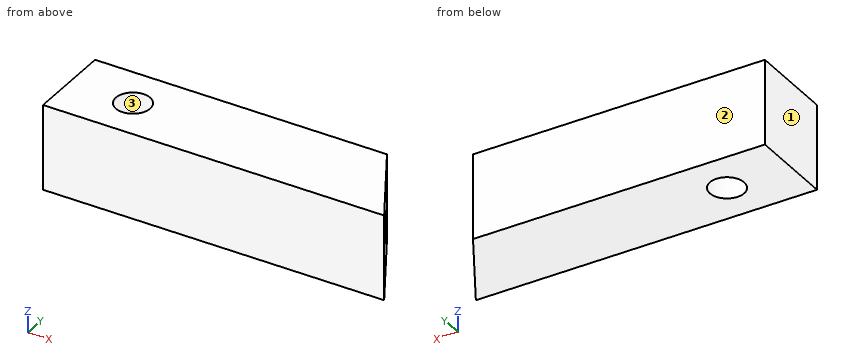
from build123d import *

# Parameters (mm, degrees)
SKETCH1_W                  = 12.7
SKETCH1_H                  = 12.7
BOSS_EXTRUDE1_DEPTH        = 50.8
F_10_32_TAPPED_HOLE1_D     = 4.0386
F_10_32_TAPPED_HOLE1_DEPTH = 25.4
F_10_32_TAPPED_HOLE1_TIP   = 1.213317848
CUT_EXTRUDE1_DEPTH         = 13.7
F_10_CLEARANCE_HOLE1_D     = 5.1054


with BuildPart() as part:
    # Sketch1 → Boss-Extrude1 (new body)
    with BuildSketch(Plane(origin=(0, 0, 0), x_dir=(0, 0, -1), z_dir=(1, 0, 0))):
        with Locations((6.35, 6.35)):
            Rectangle(SKETCH1_W, SKETCH1_H)
    extrude(amount=BOSS_EXTRUDE1_DEPTH)

    # #10-32 Tapped Hole1
    with Locations(Plane(origin=(50.8, 6.35, -6.35), x_dir=(0, 0, 1), z_dir=(1, 0, 0))):
        with Locations((0, 0)):
            Hole(F_10_32_TAPPED_HOLE1_D / 2, depth=F_10_32_TAPPED_HOLE1_DEPTH)
            with Locations((0, 0, -(F_10_32_TAPPED_HOLE1_DEPTH + F_10_32_TAPPED_HOLE1_TIP / 2))):  # 118° drill point
                Cone(0, F_10_32_TAPPED_HOLE1_D / 2, F_10_32_TAPPED_HOLE1_TIP, mode=Mode.SUBTRACT)

    # Sketch3 → Cut-Extrude1 (cut, through all)
    with BuildSketch(Plane.XY):
        Polygon((43.467651581, 12.7), (50.8, 0), (50.8, 12.7), align=None)
    extrude(amount=-CUT_EXTRUDE1_DEPTH, mode=Mode.SUBTRACT)

    # #10 Clearance Hole1 (through all)
    with Locations(Plane(origin=(9.525, 6.35, 0), x_dir=(1, 0, 0), z_dir=(0, 0, 1))):
        with Locations((0, 0)):
            Hole(F_10_CLEARANCE_HOLE1_D / 2)


solid = part.part
Can you work these out from the model? Positions are in its coordinate system, mm. Face numbers are marked on the shaded views. Give positions to 0.01 mm unless a question says otherwise; leave off trailing zeros. Write each loop counter-clockwise with the first axis right and the second up, starting at its lowest first coordinate (ties: lowest second). Pieces come first, ordered by that corner, then holes. Notation, with made-up numbers: (82, 54.25) -> (108, 54.25) arc R12 ccw to (108, 70.25) -> close; hole circle Ø3 at (-8, -6.75). An arc over 180 degrees is marked (long way). Answer as a JSON object with one key per item and string values. Group by question number.
Item 1: Suppose I cut it at C-C (x = 35.5). Please give me the cut outline in (y, z), plus the area to 3 significant figures.
Item 2: Suppose I cut it at A-A (x = 7.5). Please give me the cut outline in (y, z).
Item 3: Please list where these lines run through material, in increasing order: line 1 (Y direction, x = 36, z = -6.35); line 2 (Y direction, x = 28, z = -5); line 3 (Y direction, x = 45.5, z = -2.5). Write a range as [from, to].
Item 4: Suppose I cut it at B-B (z = -3.5). Please give me the cut outline in (x, y) (3 decimals), plus the area to 3 significant figures.
Item 5: I'm going to push a flat-ended pin straight in: P1, Ø3, axis at y = 9.5, z = -5, coming from the +X side. Where does the tip first touch, or does it pass through?
Item 6: Suppose I cut it at D-D (y = 10). Please give me the cut outline in (x, z), plus the area to 3 significant figures.
Item 7: We'd pull the mould along X, two halves only. Please class the marked faces 1, 2 and 3: +X half, -X half, draft (parallel to the pull), parting line (faces both ways), or undercut.
Findings:
{
 "1": {"outline": "(0, -12.7) -> (12.7, -12.7) -> (12.7, 0) -> (0, 0) -> close; hole circle Ø4.04 at (6.35, -6.35)", "area": "148 mm²"},
 "2": {"outline": "(0, -12.7) -> (4.8, -12.7) -> (4.8, 0) -> (0, 0) -> close; (7.9, -12.7) -> (12.7, -12.7) -> (12.7, 0) -> (7.9, 0) -> close"},
 "3": {"line 1": "y = [0, 4.33], [8.37, 12.7]", "line 2": "y = [0, 4.85], [7.85, 12.7]", "line 3": "y = [0, 9.18]"},
 "4": {"outline": "(0, 0) -> (50.8, 0) -> (43.468, 12.7) -> (0, 12.7) -> close; hole circle Ø5.105 at (9.525, 6.35)", "area": "578 mm²"},
 "5": {"P1": "stops at x = 46.18"},
 "6": {"outline": "(0, -12.7) -> (45.03, -12.7) -> (45.03, 0) -> (0, 0) -> close", "area": "572 mm²"},
 "7": {"face 1": "-X half", "face 2": "draft", "face 3": "undercut"}
}
